Check sheet for the modelled part. Datum: model origin and axes. Units: mm. A direction names the side the tool comes from. Give positions to 0.01 mm unless a question says otherwise; leave off trailing zeros. Loops run counter-clockwise (first coordinate to the right, second up) from the corner with the lowest first, then second, coordinate; pieces in that order, holes last. Notation, with made-up numbers: (84, 25.25) - (136, 25.25) arc R17 ccw to (136, 45.25) - close; hole circle Ø10 at (84, 17). An arc over 180 degrees is marked (long way). Answer in a Markdown table with one row per item. Add a question column.
(1) Draft check along Z on faces 1 (the face through (1.3, 0, 4.1)), 2 (the face through (-0.1, 3, 4.3)), 3 (the face through (7.964, 8.409, -2.508)). Enter one of: released by +Z, released by -Z, zero draft, split by the parting line, or undercut.
(2) Sectioned sample at B-B on x = 0. Enter the section's corners in (y, z).
(3) Sectioned sample at D-D on y = 11.75. Enter the section's corners in (x, z), then the cut area to 3 significant figures.
(4) Thickness scan on L1, parallel to X at y = 5.5, z = 0; L2, parallel to X at y = 1, z = -3.25; L3, parallel to Z at x = 7.05, y = 9. Record the ranges inside material, lowest first.
(5) Sectioned sample at A-A on z = 0. Enter the section's corners in (x, y).
(6) Go/stop test with flat-tipped pins: P1, Ø3, axis at x = -1, z = -2, coming from the +Y side; P2, Ø9.5, axis at x = 0, z = 0, coming from the +Y side; P3, Ø6, axis at y = 11.5, z = 4.5, coming from the +X side; P4, Ø2, axis at y = 12, z = 5, coming from the +X side. Record where each tip stops, or that it passes through.
(7) Set-up check for faces 4 (the face through (-7.409, 9.843, 0.111)), 5 (the face through (6.248, 9.084, -1.967)): record each of +Z, -Z, +X, -X, +Y, -Y from which the full face is reachable in a straight line by a thin tool's end or side.
from build123d import *

# Parameters (mm, degrees)
SKETCH1_R               = 8.35
BOSS_EXTRUDE1_DEPTH     = 15
SKETCH2_R               = 6.55
CUT_EXTRUDE1_DEPTH      = 12
SKETCH3_R               = 0.85
CUT_EXTRUDE2_DEPTH      = 9.35
CUT_EXTRUDE2_DEPTH_BACK = 9.35
SKETCH4_R               = 4.15
CUT_EXTRUDE3_DEPTH      = 16.0000001
CHAMFER1_SIZE           = 2


with BuildPart() as part:
    # Sketch1 → Boss-Extrude1 (new body)
    with BuildSketch(Plane(origin=(0, 0, 0), x_dir=(1, 0, 0), z_dir=(0, 1, 0))):
        Circle(SKETCH1_R)
    extrude(amount=BOSS_EXTRUDE1_DEPTH)

    # Sketch2 → Cut-Extrude1 (cut)
    with BuildSketch(Plane(origin=(0, 15, 0), x_dir=(1, 0, 0), z_dir=(0, 1, 0))):
        Circle(SKETCH2_R)
    extrude(amount=-CUT_EXTRUDE1_DEPTH, mode=Mode.SUBTRACT)

    # Sketch3 → Cut-Extrude2 (cut, two sides)
    with BuildSketch(Plane(origin=(0, 0, 0), x_dir=(0, 0, -1), z_dir=(1, 0, 0))) as cut_extrude2_sk:
        with Locations((0, 9)):
            Circle(SKETCH3_R)
    extrude(amount=CUT_EXTRUDE2_DEPTH, mode=Mode.SUBTRACT)
    extrude(cut_extrude2_sk.sketch, amount=-CUT_EXTRUDE2_DEPTH_BACK, mode=Mode.SUBTRACT)

    # Sketch4 → Cut-Extrude3 (cut, through all)
    with BuildSketch(Plane.XZ):
        Circle(SKETCH4_R)
    extrude(amount=-CUT_EXTRUDE3_DEPTH, mode=Mode.SUBTRACT)

    # Chamfer1
    chamfer1_edges = [part.edges().sort_by_distance(p)[0] for p in [
        (-8.35, 0, 0),
    ]]
    chamfer(chamfer1_edges, length=CHAMFER1_SIZE)


solid = part.part
Reply:
| question | item | result |
|---|---|---|
| 1 | face 1 | zero draft |
| 1 | face 2 | undercut |
| 1 | face 3 | split by the parting line |
| 2 | outline | (0, -6.35) - (2, -8.35) - (15, -8.35) - (15, -6.55) - (3, -6.55) - (3, -4.15) - (0, -4.15) - close; (0, 4.15) - (3, 4.15) - (3, 6.55) - (15, 6.55) - (15, 8.35) - (2, 8.35) - (0, 6.35) - close |
| 3 | outline | circle Ø16.7 at (0, 0); hole circle Ø13.1 at (0, 0) |
| 3 | area | 84.3 mm^2 |
| 4 | L1 | -8.35 to -6.55, 6.55 to 8.35 |
| 4 | L2 | -6.59 to -2.58, 2.58 to 6.59 |
| 4 | L3 | -4.47 to -0.85, 0.85 to 4.47 |
| 5 | outline | (-8.35, 2) - (-6.35, 0) - (-4.15, 0) - (-4.15, 3) - (-6.55, 3) - (-6.55, 8.15) - (-8.35, 8.15) - close; (-8.35, 9.85) - (-6.55, 9.85) - (-6.55, 15) - (-8.35, 15) - close; (4.15, 0) - (6.35, 0) - (8.35, 2) - (8.35, 8.15) - (6.55, 8.15) - (6.55, 3) - (4.15, 3) - close; (6.55, 9.85) - (8.35, 9.85) - (8.35, 15) - (6.55, 15) - close |
| 6 | P1 | through |
| 6 | P2 | y = 3 |
| 6 | P3 | x = 8.21 |
| 6 | P4 | x = 7.33 |
| 7 | face 4 | +X, -X |
| 7 | face 5 | +Y |
